```python
from build123d import *

# Parameters (mm, degrees)
F0_R     = 100.457
F1_DEPTH = 175.26
F2_DEPTH = 19.05
F4_DEPTH = 47.625


with BuildPart() as f1:
    # F0 (on Top) → F1 (new body)
    with BuildSketch(Plane.XY):
        Circle(F0_R)
        with BuildLine():
            ThreePointArc((4.7600731087, 74.4477794433), (52.7500244552, 52.7500244552), (74.4477794433, 4.7600731087))
            ThreePointArc((74.4477794433, 4.7600731087), (77.9132127685, 3.420921232), (79.3623, 0))
            ThreePointArc((79.3623, 0), (77.9132127685, -3.420921232), (74.4477794433, -4.7600731087))
            ThreePointArc((74.4477794433, -4.7600731087), (52.7500244552, -52.7500244552), (4.7600731087, -74.4477794433))
            ThreePointArc((4.7600731087, -74.4477794433), (4.7618932385, -74.5237800364), (4.7625, -74.5998))
            ThreePointArc((4.7625, -74.5998), (-0.0760199636, -79.3616932385), (-4.7600731087, -74.4477794433))
            ThreePointArc((-4.7600731087, -74.4477794433), (-52.7500244552, -52.7500244552), (-74.4477794433, -4.7600731087))
            ThreePointArc((-74.4477794433, -4.7600731087), (-79.3623, 0), (-74.4477794433, 4.7600731087))
            ThreePointArc((-74.4477794433, 4.7600731087), (-52.7500244552, 52.7500244552), (-4.7600731087, 74.4477794433))
            ThreePointArc((-4.7600731087, 74.4477794433), (-0.0760199636, 79.3616932385), (4.7625, 74.5998))
            ThreePointArc((4.7625, 74.5998), (4.7618932385, 74.5237800364), (4.7600731087, 74.4477794433))
        make_face(mode=Mode.SUBTRACT)
        with BuildLine():
            ThreePointArc((-74.4477794433, -4.7600731087), (-74.5998, 0), (-74.4477794433, 4.7600731087))
            ThreePointArc((-74.4477794433, 4.7600731087), (-79.3623, 0), (-74.4477794433, -4.7600731087))
        make_face()
        with BuildLine():
            ThreePointArc((-69.8373, 0), (-71.178878768, 3.3134127685), (-74.4477794433, 4.7600731087))
            ThreePointArc((-74.4477794433, 4.7600731087), (-74.5998, 0), (-74.4477794433, -4.7600731087))
            ThreePointArc((-74.4477794433, -4.7600731087), (-71.178878768, -3.3134127685), (-69.8373, 0))
        make_face()
        with BuildLine():
            ThreePointArc((-4.7600731087, 74.4477794433), (0, 74.5998), (4.7600731087, 74.4477794433))
            ThreePointArc((4.7600731087, 74.4477794433), (4.7618932385, 74.5237800364), (4.7625, 74.5998))
            ThreePointArc((4.7625, 74.5998), (-0.0760199636, 79.3616932385), (-4.7600731087, 74.4477794433))
        make_face()
        with BuildLine():
            ThreePointArc((-4.7600731087, 74.4477794433), (0, 69.8373), (4.7600731087, 74.4477794433))
            ThreePointArc((4.7600731087, 74.4477794433), (0, 74.5998), (-4.7600731087, 74.4477794433))
        make_face()
        with BuildLine():
            ThreePointArc((74.4477794433, -4.7600731087), (74.561785175, -2.38125), (74.5998, 0))
            ThreePointArc((74.5998, 0), (74.561785175, 2.38125), (74.4477794433, 4.7600731087))
            ThreePointArc((74.4477794433, 4.7600731087), (69.8373, 0), (74.4477794433, -4.7600731087))
        make_face()
        with BuildLine():
            ThreePointArc((74.4477794433, 4.7600731087), (74.561785175, 2.38125), (74.5998, 0))
            ThreePointArc((74.5998, 0), (74.561785175, -2.38125), (74.4477794433, -4.7600731087))
            ThreePointArc((74.4477794433, -4.7600731087), (77.9132127685, -3.420921232), (79.3623, 0))
            ThreePointArc((79.3623, 0), (77.9132127685, 3.420921232), (74.4477794433, 4.7600731087))
        make_face()
        with BuildLine():
            ThreePointArc((4.7625, -74.5998), (4.7618932385, -74.5237800364), (4.7600731087, -74.4477794433))
            ThreePointArc((4.7600731087, -74.4477794433), (0, -74.5998), (-4.7600731087, -74.4477794433))
            ThreePointArc((-4.7600731087, -74.4477794433), (-0.0760199636, -79.3616932385), (4.7625, -74.5998))
        make_face()
        with BuildLine():
            ThreePointArc((74.4477794433, -4.7600731087), (69.8373, 0), (74.4477794433, 4.7600731087))
            ThreePointArc((74.4477794433, 4.7600731087), (52.7500244552, 52.7500244552), (4.7600731087, 74.4477794433))
            ThreePointArc((4.7600731087, 74.4477794433), (0, 69.8373), (-4.7600731087, 74.4477794433))
            ThreePointArc((-4.7600731087, 74.4477794433), (-52.7500244552, 52.7500244552), (-74.4477794433, 4.7600731087))
            ThreePointArc((-74.4477794433, 4.7600731087), (-71.178878768, 3.3134127685), (-69.8373, 0))
            ThreePointArc((-69.8373, 0), (-71.178878768, -3.3134127685), (-74.4477794433, -4.7600731087))
            ThreePointArc((-74.4477794433, -4.7600731087), (-52.7500244552, -52.7500244552), (-4.7600731087, -74.4477794433))
            ThreePointArc((-4.7600731087, -74.4477794433), (0, -69.8373), (4.7600731087, -74.4477794433))
            ThreePointArc((4.7600731087, -74.4477794433), (52.7500244552, -52.7500244552), (74.4477794433, -4.7600731087))
        make_face()
        with BuildLine():
            ThreePointArc((-4.7600731087, -74.4477794433), (0, -74.5998), (4.7600731087, -74.4477794433))
            ThreePointArc((4.7600731087, -74.4477794433), (0, -69.8373), (-4.7600731087, -74.4477794433))
        make_face()
    extrude(amount=F1_DEPTH)

    # F0 (on Top) → F2 (cut)
    with BuildSketch(Plane.XY):
        with BuildLine():
            ThreePointArc((-69.8373, 0), (-71.178878768, 3.3134127685), (-74.4477794433, 4.7600731087))
            ThreePointArc((-74.4477794433, 4.7600731087), (-74.5998, 0), (-74.4477794433, -4.7600731087))
            ThreePointArc((-74.4477794433, -4.7600731087), (-71.178878768, -3.3134127685), (-69.8373, 0))
        make_face()
        with BuildLine():
            ThreePointArc((-74.4477794433, -4.7600731087), (-74.5998, 0), (-74.4477794433, 4.7600731087))
            ThreePointArc((-74.4477794433, 4.7600731087), (-79.3623, 0), (-74.4477794433, -4.7600731087))
        make_face()
        with BuildLine():
            ThreePointArc((-4.7600731087, 74.4477794433), (0, 69.8373), (4.7600731087, 74.4477794433))
            ThreePointArc((4.7600731087, 74.4477794433), (0, 74.5998), (-4.7600731087, 74.4477794433))
        make_face()
        with BuildLine():
            ThreePointArc((-4.7600731087, 74.4477794433), (0, 74.5998), (4.7600731087, 74.4477794433))
            ThreePointArc((4.7600731087, 74.4477794433), (4.7618932385, 74.5237800364), (4.7625, 74.5998))
            ThreePointArc((4.7625, 74.5998), (-0.0760199636, 79.3616932385), (-4.7600731087, 74.4477794433))
        make_face()
        with BuildLine():
            ThreePointArc((74.4477794433, -4.7600731087), (74.561785175, -2.38125), (74.5998, 0))
            ThreePointArc((74.5998, 0), (74.561785175, 2.38125), (74.4477794433, 4.7600731087))
            ThreePointArc((74.4477794433, 4.7600731087), (69.8373, 0), (74.4477794433, -4.7600731087))
        make_face()
        with BuildLine():
            ThreePointArc((74.4477794433, 4.7600731087), (74.561785175, 2.38125), (74.5998, 0))
            ThreePointArc((74.5998, 0), (74.561785175, -2.38125), (74.4477794433, -4.7600731087))
            ThreePointArc((74.4477794433, -4.7600731087), (77.9132127685, -3.420921232), (79.3623, 0))
            ThreePointArc((79.3623, 0), (77.9132127685, 3.420921232), (74.4477794433, 4.7600731087))
        make_face()
        with BuildLine():
            ThreePointArc((4.7625, -74.5998), (4.7618932385, -74.5237800364), (4.7600731087, -74.4477794433))
            ThreePointArc((4.7600731087, -74.4477794433), (0, -74.5998), (-4.7600731087, -74.4477794433))
            ThreePointArc((-4.7600731087, -74.4477794433), (-0.0760199636, -79.3616932385), (4.7625, -74.5998))
        make_face()
        with BuildLine():
            ThreePointArc((-4.7600731087, -74.4477794433), (0, -74.5998), (4.7600731087, -74.4477794433))
            ThreePointArc((4.7600731087, -74.4477794433), (0, -69.8373), (-4.7600731087, -74.4477794433))
        make_face()
    extrude(amount=F2_DEPTH, mode=Mode.SUBTRACT)

    # F3 (on face) → F4 (join)
    with BuildSketch(Plane.XY):
        with BuildLine():
            ThreePointArc((2.3876, -10.8529729793), (8.6608273638, -6.962594748), (11.1125, 0))
            ThreePointArc((11.1125, 0), (-6.962594748, 8.6608273638), (-2.3876, -10.8529729793))
            Line((-2.3876, -10.8529729793), (-2.3876, -8.4582))
            Line((-2.3876, -8.4582), (2.3876, -8.4582))
            Line((2.3876, -8.4582), (2.3876, -10.8529729793))
        make_face()
    extrude(amount=-F4_DEPTH)


solid = f1.part
```
The model under review builds one solid part; all positions refer to its coordinate system, in mm. A direction names the side the tool comes from. Round coordinates to 2 decimals unless told otherwise and drop trailing zeros. Order: outer loops, then holes, each group sorted by start corner. A loop starts at its lowest first (then second) coordinate and runs counter-clockwise, first axis right, second up.
(1) Take a section at C-C, the plane y = -59.5. State the section outline as (x, z) points.
Working result:
outline: (-80.94, 0) - (80.94, 0) - (80.94, 175.26) - (-80.94, 175.26) - close
(2) Mouldability with a two-part tool opening along X and no side actions: class faces 3 (the face through (95.82, 30.17, 86.4)), 4 (the face through (-1, 1, 175.26)), 5 (the face through (75, 0, 19.05)) as released by +X, released by -X, zero draft, split by the parting line, or undercut.
Working result:
face 3: split by the parting line
face 4: zero draft
face 5: undercut
(3) Tool access review of faces 1 (the face through (0, -75, 19.05)), 2 (the face through (0, 0, -47.625)): name each direction out of +Z, -Z, +X, -X, +Y, -Y from which nothing blocks a thin tool from reaching the whole face with its end or side.
Working result:
face 1: -Z
face 2: -Z, +X, -X, +Y, -Y
(4) Take a section at A-A, the plane z = 56.5. State the section outline as (x, y) points.
Working result:
outline: circle Ø200.91 at (0, 0)
(5) Take a section at B-B, the plane x = -15. State the section outline as (y, z) points.
Working result:
outline: (-99.33, 0) - (99.33, 0) - (99.33, 175.26) - (-99.33, 175.26) - close
(6) Wall thickness on L1, parallel to Y at x = 0, z = 15; L2, parallel to Z at x = -81, y = 39; L3, parallel to X at y = 27.5, z = 155.5: over which ranges is each line inside the solid? List them lowest first.
Working result:
L1: y = -100.46 to -79.36, -69.84 to 69.84, 79.36 to 100.46
L2: z = 0 to 175.26
L3: x = -96.62 to 96.62
(7) For P1, Ø3, axis at x = 0.5, y = -75, coming from the -Z side; P2, Ø1.2, axis at y = -10, z = -17.5, coming from the +X side; P3, Ø1.2, axis at y = -10, z = -23, coming from the -X side, all flat-tipped, find the tip position at first contact; note any pin that passes through.
Working result:
P1: stops at z = 19.05
P2: stops at x = 5.93
P3: stops at x = -5.93
